Build history of the part. All positions in model axes, mm. Face numbers are marked on the shaded views. A direction names the side the tool comes from. Give positions to 0.01 mm unless a question says otherwise; leave off trailing zeros. Order: outer loops, then holes, each group sorted by start corner. A loop starts at its lowest first (then second) coordinate and runs counter-clockwise, first axis right, second up. Notation, with made-up numbers: (59.5, -18.5) -> (115.5, -18.5) arc R25 ccw to (115.5, -0.5) -> close; hole circle Ø8 at (82, 55). An arc over 180 degrees is marked (long way). One line per item, written item: value. Start each with the question number.
(1) Saw through at B-B on y = 14. Give the cut face in (x, z).
(2) Saw through at A-A on x = 0. Give the cut face in (y, z).
(3) Saw through at C-C on z = -5. Give the cut face in (x, y), plus the area to 3 significant figures.
(4) Pin check, flat tips, straight feed: pin 1 (2.5 mm diameter, centred on x = 17, z = -13, fed in from +Y); pin 2 (0.9 mm diameter, centred on x = 16.5, z = 12.5, fed in from +Y); pin 3 (1.6 mm diameter, centred on x = -20, y = 38.5, fed in from -Z). Stop position of each tip, or through.
(5) Probe line 1 (Z direction, x = -7, y = 9.5); line 2 (X direction, y = 46.5, z = -14); line 3 (Y direction, x = 10.5, z = -8.5). List the from-to ranges inside material, lowest first.
(6) Saw through at D-D on y = 64.5. Give the cut face in (x, z).
(7) Which spindle directions (+Z, -Z, +X, -X, +Y, -Y) get a long thin tool onto all of the face, cutting with end or side? Do the marked faces 1, 2 and 3. Say none if no direction does.
(8) Two-plate mould, pull along Y, no slides. Class the marked faces 4, 5 and 6: +Y half, -Y half, draft (parallel to the pull), parting line (faces both ways), or undercut.
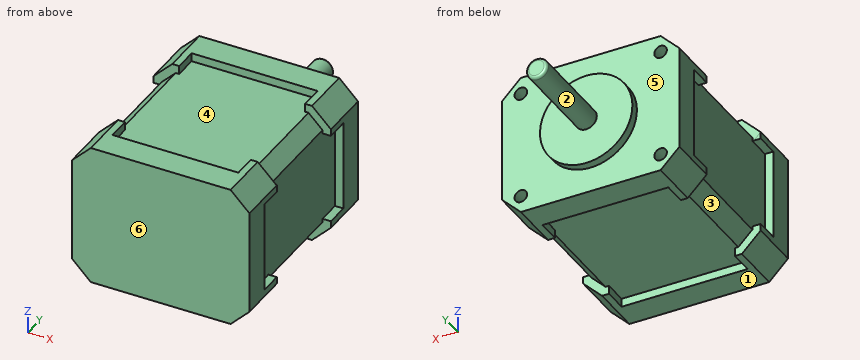
```python
from build123d import *

# Parameters (mm, degrees)
SKETCH1_W           = 42.3
SKETCH1_H           = 33.84
BOSS_EXTRUDE1_DEPTH = 48
SKETCH2_R           = 11.009712126
BOSS_EXTRUDE2_DEPTH = 2
CHAMFER1_SIZE       = 4.5
CHAMFER2_SIZE       = 4.5
CHAMFER3_SIZE       = 4.5
CHAMFER4_SIZE       = 4.5
SKETCH3_R           = 2.52352428
BOSS_EXTRUDE3_DEPTH = 22
SKETCH4_R           = 1.5
CUT_EXTRUDE1_DEPTH  = 4.5
FILLET4_R           = 0.7
SKETCH5_W           = 30
SKETCH5_H           = 35
SKETCH5_W_2         = 1.65
SKETCH5_H_2         = 24
CUT_EXTRUDE2_DEPTH  = 2
SKETCH6_W           = 6.363961031
SKETCH6_H           = 24
CUT_EXTRUDE4_DEPTH  = 2
SKETCH8_W           = 21.54
SKETCH8_H           = 5.5
SKETCH8_H_2         = 23.916619391
SKETCH8_W_2         = 1.65
CUT_EXTRUDE5_DEPTH  = 2
SKETCH9_W           = 6.363961031
SKETCH9_H           = 23.916619391
CUT_EXTRUDE7_DEPTH  = 2
SKETCH10_W          = 33.3
SKETCH10_H          = 23.916619391
CUT_EXTRUDE8_DEPTH  = 2
SKETCH11_W          = 30
SKETCH11_H          = 35
CUT_EXTRUDE10_DEPTH = 2
SKETCH12_W          = 6.363961031
SKETCH12_H          = 23.916619391
CUT_EXTRUDE11_DEPTH = 2
SKETCH13_W          = 6.363961031
SKETCH13_H          = 24
CUT_EXTRUDE12_DEPTH = 2
SKETCH14_W          = 21.54
SKETCH14_H          = 5.5
SKETCH14_H_2        = 23.916619391
SKETCH14_H_3        = 5.583380609
SKETCH14_W_2        = 1.65
CUT_EXTRUDE13_DEPTH = 2


with BuildPart() as part:
    # Sketch1 → Boss-Extrude1 (new body)
    with BuildSketch(Plane(origin=(0, 0, 0), x_dir=(1, 0, 0), z_dir=(0, 1, 0))):
        Rectangle(SKETCH1_W, SKETCH1_H)
    extrude(amount=BOSS_EXTRUDE1_DEPTH)

    # Sketch2 → Boss-Extrude2 (add)
    with BuildSketch(Plane(origin=(0, 48, 0), x_dir=(1, 0, 0), z_dir=(0, 1, 0))):
        with Locations(Location((0, 0, 0), (0, 0, 270))):
            Circle(SKETCH2_R)
    extrude(amount=BOSS_EXTRUDE2_DEPTH)

    # Chamfer1
    chamfer1_edges = [part.edges().sort_by_distance(p)[0] for p in [
        (21.15, 24, 16.92),
    ]]
    chamfer(chamfer1_edges, length=CHAMFER1_SIZE)

    # Chamfer2
    chamfer2_edges = [part.edges().sort_by_distance(p)[0] for p in [
        (-21.15, 24, 16.92),
    ]]
    chamfer(chamfer2_edges, length=CHAMFER2_SIZE)

    # Chamfer3
    chamfer3_edges = [part.edges().sort_by_distance(p)[0] for p in [
        (21.15, 24, -16.92),
    ]]
    chamfer(chamfer3_edges, length=CHAMFER3_SIZE)

    # Chamfer4
    chamfer4_edges = [part.edges().sort_by_distance(p)[0] for p in [
        (-21.15, 24, -16.92),
    ]]
    chamfer(chamfer4_edges, length=CHAMFER4_SIZE)

    # Sketch3 → Boss-Extrude3 (add)
    with BuildSketch(Plane(origin=(0, 50, 0), x_dir=(1, 0, 0), z_dir=(0, 1, 0))):
        with Locations(Location((0, 0, 0), (0, 0, 270))):
            Circle(SKETCH3_R)
    extrude(amount=BOSS_EXTRUDE3_DEPTH)

    # Sketch4 → Cut-Extrude1 (cut)
    with BuildSketch(Plane(origin=(0, 48, 0), x_dir=(1, 0, 0), z_dir=(0, 1, 0))):
        with Locations(Location((-16.65, -12.923571429, 0), (0, 0, 270))):
            Circle(SKETCH4_R)
        with Locations(Location((-16.65, 12.923571429, 0), (0, 0, 270))):
            Circle(SKETCH4_R)
        with Locations(Location((16.65, 12.923571429, 0), (0, 0, 270))):
            Circle(SKETCH4_R)
        with Locations(Location((16.65, -12.923571429, 0), (0, 0, 270))):
            Circle(SKETCH4_R)
    extrude(amount=-CUT_EXTRUDE1_DEPTH, mode=Mode.SUBTRACT)

    # Fillet4
    fillet4_edges = [part.edges().sort_by_distance(p)[0] for p in [
        (0, 72, -2.52352428),
    ]]
    fillet(fillet4_edges, radius=FILLET4_R)

    # Sketch5 → Cut-Extrude2 (cut)
    with BuildSketch(Plane.XY.offset(16.92)):
        with Locations((0, 24)):
            Rectangle(SKETCH5_W, SKETCH5_H)
        with Locations((15.825, 24)):
            Rectangle(SKETCH5_W_2, SKETCH5_H_2)
        with Locations((-15.825, 24)):
            Rectangle(SKETCH5_W_2, SKETCH5_H_2)
    extrude(amount=-CUT_EXTRUDE2_DEPTH, mode=Mode.SUBTRACT)

    # Sketch6 → Cut-Extrude4 (cut)
    with BuildSketch(Plane(origin=(16.785, 0, 16.785), x_dir=(0.707106781186549, 0, -0.707106781186546), z_dir=(0.707106781186546, 0, 0.707106781186549))):
        with Locations((2.991061684, 24)):
            Rectangle(SKETCH6_W, SKETCH6_H)
    extrude(amount=-CUT_EXTRUDE4_DEPTH, mode=Mode.SUBTRACT)

    # Sketch8 → Cut-Extrude5 (cut)
    with BuildSketch(Plane(origin=(21.15, 0, 0), x_dir=(0, 0, -1), z_dir=(1, 0, 0))):
        with Locations((0, 38.75)):
            Rectangle(SKETCH8_W, SKETCH8_H)
        with Locations((0, 24.041690305)):
            Rectangle(SKETCH8_W, SKETCH8_H_2)
        with Locations((0, 9.333380609)):
            Rectangle(SKETCH8_W, SKETCH8_H)
        with Locations((11.595, 24.041690305)):
            Rectangle(SKETCH8_W_2, SKETCH8_H_2)
        with Locations((-11.595, 24.041690305)):
            Rectangle(SKETCH8_W_2, SKETCH8_H_2)
    extrude(amount=-CUT_EXTRUDE5_DEPTH, mode=Mode.SUBTRACT)

    # Sketch9 → Cut-Extrude7 (cut)
    with BuildSketch(Plane(origin=(16.785, 0, -16.785), x_dir=(-0.707106781186546, 0, -0.7071067811865491), z_dir=(0.7071067811865491, 0, -0.707106781186546))):
        with Locations((-2.991061684, 24.041690305)):
            Rectangle(SKETCH9_W, SKETCH9_H)
    extrude(amount=-CUT_EXTRUDE7_DEPTH, mode=Mode.SUBTRACT)

    # Sketch10 → Cut-Extrude8 (cut)
    with BuildSketch(Plane(origin=(0, 0, -16.92), x_dir=(-1, 0, 0), z_dir=(0, 0, -1))):
        with Locations((0, 24.041690305)):
            Rectangle(SKETCH10_W, SKETCH10_H)
    extrude(amount=-CUT_EXTRUDE8_DEPTH, mode=Mode.SUBTRACT)

    # Sketch11 → Cut-Extrude10 (cut)
    with BuildSketch(Plane(origin=(0, 0, -16.92), x_dir=(-1, 0, 0), z_dir=(0, 0, -1))):
        with Locations((0, 24)):
            Rectangle(SKETCH11_W, SKETCH11_H)
    extrude(amount=-CUT_EXTRUDE10_DEPTH, mode=Mode.SUBTRACT)

    # Sketch12 → Cut-Extrude11 (cut)
    with BuildSketch(Plane(origin=(-16.785, 0, -16.785), x_dir=(-0.7071067811865491, 0, 0.707106781186546), z_dir=(-0.707106781186546, 0, -0.7071067811865491))):
        with Locations((2.991061684, 24.041690305)):
            Rectangle(SKETCH12_W, SKETCH12_H)
    extrude(amount=-CUT_EXTRUDE11_DEPTH, mode=Mode.SUBTRACT)

    # Sketch13 → Cut-Extrude12 (cut)
    with BuildSketch(Plane(origin=(-16.785, 0, 16.785), x_dir=(0.7071067811865465, 0, 0.7071067811865486), z_dir=(-0.7071067811865486, 0, 0.7071067811865465))):
        with Locations((-2.991061684, 24)):
            Rectangle(SKETCH13_W, SKETCH13_H)
    extrude(amount=-CUT_EXTRUDE12_DEPTH, mode=Mode.SUBTRACT)

    # Sketch14 → Cut-Extrude13 (cut)
    with BuildSketch(Plane.ZY.offset(21.15)):
        with Locations((0, 38.75)):
            Rectangle(SKETCH14_W, SKETCH14_H)
        with Locations((0, 24.041690305)):
            Rectangle(SKETCH14_W, SKETCH14_H_2)
        with Locations((0, 9.291690305)):
            Rectangle(SKETCH14_W, SKETCH14_H_3)
        with Locations((11.595, 24.041690305)):
            Rectangle(SKETCH14_W_2, SKETCH14_H_2)
        with Locations((-11.595, 24.041690305)):
            Rectangle(SKETCH14_W_2, SKETCH14_H_2)
    extrude(amount=-CUT_EXTRUDE13_DEPTH, mode=Mode.SUBTRACT)


solid = part.part
```
Results below:
1. outline: (-19.15, -11.59) -> (-15.82, -14.92) -> (15.82, -14.92) -> (19.15, -11.59) -> (19.15, 11.59) -> (15.82, 14.92) -> (-15.82, 14.92) -> (-19.15, 11.59) -> close
2. outline: (0, -16.92) -> (6.5, -16.92) -> (6.5, -14.92) -> (41.5, -14.92) -> (41.5, -16.92) -> (48, -16.92) -> (48, -11.01) -> (50, -11.01) -> (50, -2.52) -> (71.3, -2.52) arc R0.7 ccw to (72, -1.82) -> (72, 1.82) arc R0.7 ccw to (71.3, 2.52) -> (50, 2.52) -> (50, 11.01) -> (48, 11.01) -> (48, 16.92) -> (41.5, 16.92) -> (41.5, 14.92) -> (6.5, 14.92) -> (6.5, 16.92) -> (0, 16.92) -> close
3. outline: (-21.15, 0) -> (21.15, 0) -> (21.15, 6.58) -> (19.15, 6.58) -> (19.15, 41.5) -> (21.15, 41.5) -> (21.15, 48) -> (9.81, 48) -> (9.81, 50) -> (-9.81, 50) -> (-9.81, 48) -> (-21.15, 48) -> (-21.15, 41.5) -> (-19.15, 41.5) -> (-19.15, 6.5) -> (-21.15, 6.5) -> close
3. area: 1,930 mm²
4. pin 1: stops at y = 48
4. pin 2: stops at y = 43.5
4. pin 3: stops at z = -14.37
5. line 1: z = -14.92 to 14.92
5. line 2: x = -19.57 to -17.69, -15.61 to 15.61, 17.69 to 19.57
5. line 3: y = 0 to 48
6. outline: circle Ø5.05 at (0, 0)
7. face 1: -Z, +X, -X, +Y, -Y
7. face 2: +Y
7. face 3: -Z, -X
8. face 4: undercut
8. face 5: +Y half
8. face 6: -Y half
